Geometry check sheet. Reference: drawing and pictorial views, mm from the part's lowest x, y, z. Round coordinates to 2 decimals unless told otherwise and drop trailing zeros. Order: outer loops, then holes, each group sorted by start corner. A loop starts at its lowest first (then second) coordinate and runs counter-clockwise, first axis right, second up.
(1) Go/stop test with a flat-tipped pin: pin 1 (3 mm diameter, centred on x = 9.525, z = 45.865, fed in from +Y). Record where the tip stops, or that it passes through.
(2) Sectioned sample at C-C (y = 4.5). Give the number of separate pieces and of enclosed holes in the cut face, plus the area to 3 significant figures.
(3) Sectioned sample at B-B (x = 95.25). Record the boundary of the cut face in (y, z).
(4) Sectioned sample at A-A (x = 52.39). Record the boundary of the cut face in (y, z).
(5) Material ranges on line 1 along Z through (x, y) = (95.25, 4.25); line 2 along X through (y, z) = (6, 7.5) (1 decimal); line 3 along Z through (x, y) = (52.39, 2.25), recorded low to high.
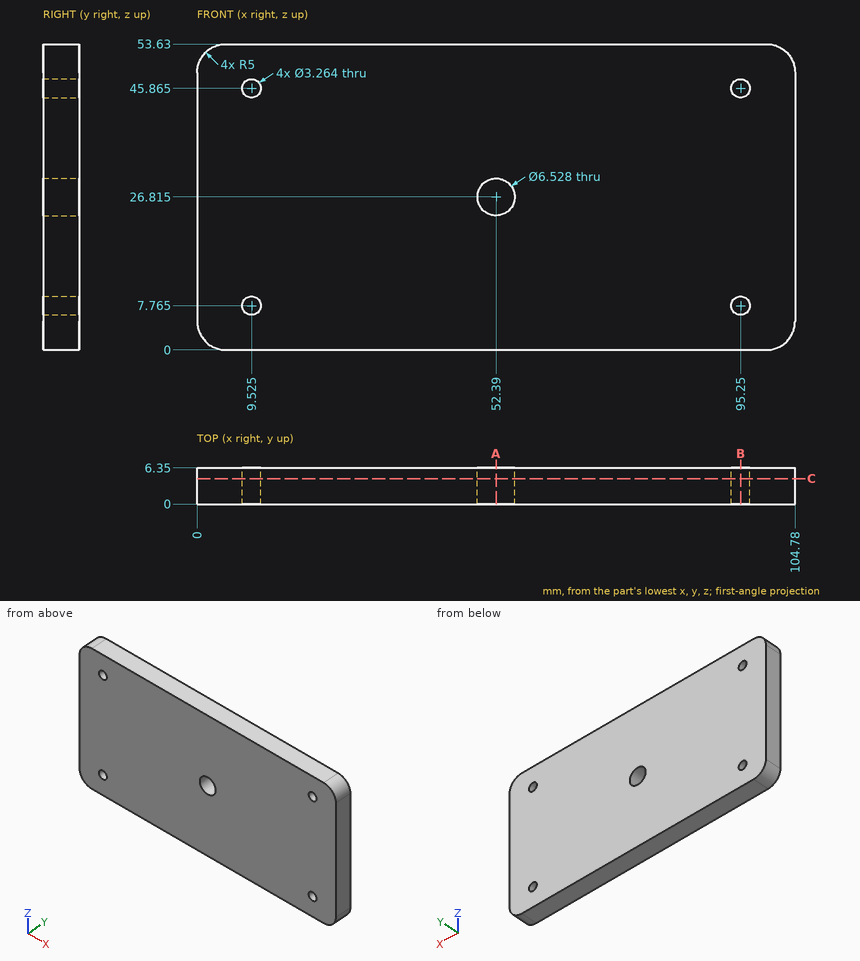
Answer below:
1. pin 1: passes through
2. separate pieces: 1
2. enclosed holes: 5
2. area: 5,530 mm2
3. outline: (0, 0) - (6.35, 0) - (6.35, 6.13) - (0, 6.13) - close; (0, 9.4) - (6.35, 9.4) - (6.35, 44.23) - (0, 44.23) - close; (0, 47.5) - (6.35, 47.5) - (6.35, 53.63) - (0, 53.63) - close
4. outline: (0, 0) - (6.35, 0) - (6.35, 23.55) - (0, 23.55) - close; (0, 30.08) - (6.35, 30.08) - (6.35, 53.63) - (0, 53.63) - close
5. line 1: z = 0 to 6.13, 9.4 to 44.23, 47.5 to 53.63
5. line 2: x = 0 to 7.9, 11.1 to 93.6, 96.9 to 104.8
5. line 3: z = 0 to 23.55, 30.08 to 53.63
